Work out the finished part from the listing and answer in its coordinate system (mm). Face numbers are marked on the shaded views. A direction names the side the tool comes from. Coordinates: 2 decimals unless noted, no trailing zeros. Write each loop counter-clockwise with the first axis right and the second up, starting at its lowest first coordinate (ties: lowest second). Pieces come first, ordered by that corner, then holes. Notation, with made-up numbers: M -15.75,59 L 4.25,59 A20 ccw 4.25,73 Z; hole C -38,-35 d4. An arc over 180 degrees is marked long. Answer as CSV lines item,"result". Start each with the question number.
(1) Find the intervals of material crossed by L1, parallel to X at y = -12, z = -19; L2, parallel to X at y = -156, z = -541.5; L3, parallel to Z at x = -135.5, y = 263, in increasing order. Write a range as [from, to].
(2) A cutting plane is placed at A-A on y = 0. Give the vertices of the cut face in (x, z), then the cut area to 3 significant figures.
(3) A cutting plane is placed at C-C on x = 0. Give the vertices of the cut face in (y, z).
(4) Flat-ended cylindrical pins translate along their axes: P1, Ø22, axis at y = -91, z = 246, coming from the +X side; P2, Ø2, axis at y = -236, z = -342.5, coming from the -X side; P3, Ø8, axis at y = -133, z = -870, coming from the +X side. Find the tip coordinate at first contact, or state that the pin passes through.
(5) A cutting plane is placed at D-D on z = 142.5. Give the vertices of the cut face in (x, y).
(6) For the marked faces 1 and 2, determine the directions among +Z, -Z, +X, -X, +Y, -Y from which every point of the face is accessible in a straight line to the end or side of a thin tool.
(7) A cutting plane is placed at B-B on z = -145.5. Give the vertices of the cut face in (x, y), then the cut area to 3 significant figures.
Solid Edge part; units mm, degrees
sketch "Sketch1" plane through (0, 0, 0) normal (0, -1, 0) x (1, 0, 0)
  line L0 (264, 0) -> (264, -1100)
  line L1 (264, -1100) -> (0, -1100)
  line L2 (0, 0) -> (0, -1100)
  line L3 (0, 0) -> (0, 264)
  line L4 (0, 264) -> (484, 264)
  line L5 (264, 0) -> (484, 264)
revolve "RevolvedProtrusion1" add sketch "Sketch1" angle 360 about axis through (0, 0, 0) along (0, 0, -1)
sketch "Sketch2" plane through (0, 0, 0) normal (0, -1, 0) x (1, 0, 0)
  line L0 (-44, 264) -> (-44, 220)
  line L1 (-44, 220) -> (44, 220)
  line L2 (44, 220) -> (44, 264)
  line L3 (44, 264) -> (0, 264)
  line L4 (0, 264) -> (-44, 264)
extrude "Cutout1" cut sketch "Sketch2" along normal up to next and the other way up to next
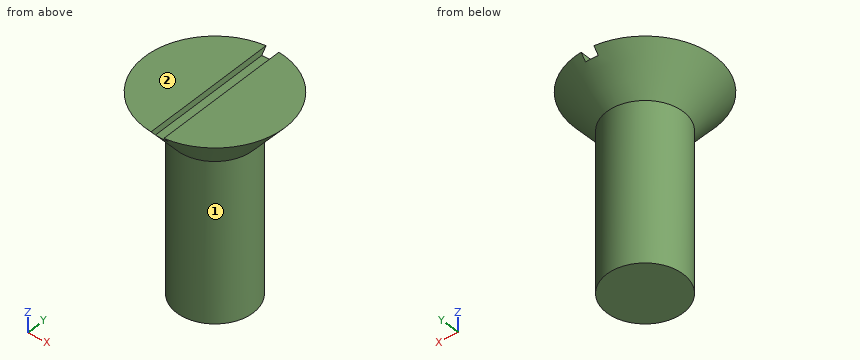
Here are the results:
1,L1,"x = [-263.73, 263.73]"
1,L2,"x = [-212.98, 212.98]"
1,L3,"z = [38.22, 264]"
2,outline,"M -484,264 L -264,0 L -264,-1100 L 264,-1100 L 264,0 L 484,264 L 44,264 L 44,220 L -44,220 L -44,264 Z"
2,area,"774,000 mm^2"
3,outline,"M -447.33,220 L -264,0 L -264,-1100 L 264,-1100 L 264,0 L 447.33,220 Z"
4,P1,"stops at x = 469.66"
4,P2,"stops at x = -120.3"
4,P3,"stops at x = 230.34"
5,outline,"C 0,0 d765.5"
6,face 1,"-Z"
6,face 2,"+Z, +X, -X, +Y, -Y"
7,outline,"C 0,0 d528"
7,area,"219,000 mm^2"
